Could you check a few things on this model? Use its own coordinates, in mm. Face numbers are marked on the shaded views. A direction names the side the tool comes from. Coordinates: 2 decimals unless noted, no trailing zeros. Loops run counter-clockwise (first coordinate to the right, second up) from the corner with the lowest first, then second, coordinate; pieces in that order, holes last.
from build123d import *

# Parameters (mm, degrees)
BOSS_EXTRUDE1_DEPTH = 215.9
BOSS_EXTRUDE2_DEPTH = 50.8
SKETCH4_W           = 19.05
SKETCH4_H           = 9.525
CUT_EXTRUDE1_DEPTH  = 31.1625
SKETCH3_R           = 3.175
BOSS_EXTRUDE3_DEPTH = 19.05


with BuildPart() as part:
    # Sketch1 → Boss-Extrude1 (new body, symmetric)
    with BuildSketch(Plane.XY):
        with BuildLine():
            Line((-19.05, -12.7), (19.05, -12.7))
            ThreePointArc((19.05, -12.7), (23.540128061, -10.840128061), (25.4, -6.35))
            Line((25.4, -6.35), (25.4, 6.35))
            ThreePointArc((25.4, 6.35), (23.540128061, 10.840128061), (19.05, 12.7))
            Line((19.05, 12.7), (-19.05, 12.7))
            ThreePointArc((-19.05, 12.7), (-23.540128061, 10.840128061), (-25.4, 6.35))
            Line((-25.4, 6.35), (-25.4, -6.35))
            ThreePointArc((-25.4, -6.35), (-23.540128061, -10.840128061), (-19.05, -12.7))
        make_face()
        with BuildLine():
            Line((-19.05, 11.049), (19.05, 11.049))
            ThreePointArc((19.05, 11.049), (22.372694765, 9.672694765), (23.749, 6.35))
            Line((23.749, 6.35), (23.749, -6.35))
            ThreePointArc((23.749, -6.35), (22.372694765, -9.672694765), (19.05, -11.049))
            Line((19.05, -11.049), (-19.05, -11.049))
            ThreePointArc((-19.05, -11.049), (-22.372694765, -9.672694765), (-23.749, -6.35))
            Line((-23.749, -6.35), (-23.749, 6.35))
            ThreePointArc((-23.749, 6.35), (-22.372694765, 9.672694765), (-19.05, 11.049))
        make_face(mode=Mode.SUBTRACT)
    extrude(amount=BOSS_EXTRUDE1_DEPTH, both=True)

    # Sketch2 → Boss-Extrude2 (add, through all)
    with BuildSketch(Plane(origin=(25.4, 0, 0), x_dir=(0, 0, -1), z_dir=(1, 0, 0))):
        with BuildLine():
            Line((203.2, -12.7), (203.2, -17.4625))
            Line((203.2, -17.4625), (220.6625, -17.4625))
            ThreePointArc((220.6625, -17.4625), (224.030096045, -9.332403955), (215.9, -12.7))
            Line((215.9, -12.7), (203.2, -12.7))
        make_face()
    extrude(amount=-BOSS_EXTRUDE2_DEPTH)

    # Sketch4 → Cut-Extrude1 (cut, through all)
    with BuildSketch(Plane.XZ.offset(17.4625)):
        with Locations((0, -220.6625)):
            Rectangle(SKETCH4_W, SKETCH4_H)
    extrude(amount=-CUT_EXTRUDE1_DEPTH, mode=Mode.SUBTRACT)

    # Sketch3 → Boss-Extrude3 (add, symmetric)
    with BuildSketch(Plane(origin=(0, 0, 0), x_dir=(0, 0, -1), z_dir=(1, 0, 0))):
        with Locations((220.6625, -12.7)):
            Circle(SKETCH3_R)
    extrude(amount=BOSS_EXTRUDE3_DEPTH, both=True)


solid = part.part
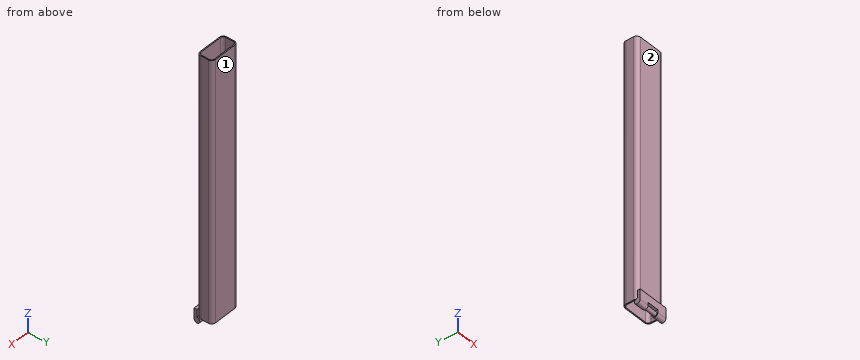
1) If I drill on L1, parallel to X at y = -4, z = -165; L2, parallel to Y at x = -10, z = 74; L3, parallel to Z at x = -0.5, y = -13, over which ranges is the centre line in solid material (lowest first)?
2) Imagine slicing it at A-A on z = 41. List the corners of the cut face in (x, y) for me, plus the area to 3 significant figures.
3) Will these pins go through, and if not, where does the flat tip stop? pin 1 (1.4 mm diameter, centred on x = -12.5, y = -15, fed in from +Z); pin 2 (19 mm diameter, centred on x = -3.5, z = 65, fed in from -Y); pin 3 (5 mm diameter, centred on x = -23, z = -210, fed in from +Y).
4) Imagine slicing it at B-B on x = -4. State how many separate pieces and enclosed holes the cut face has, plus the area to 3 significant figures.
5) For the marked faces 1 and 2, which set-ups out of +Z, -Z, +X, -X, +Y, -Y let a thin tool reach every point of the face, with its end or its side?
Solved:
1. L1: x = -25.4 to -23.75, 23.75 to 25.4
1. L2: y = -12.7 to -11.05, 11.05 to 12.7
1. L3: z = -223.82 to -217.5, -215.9 to -203.2
2. outline: (-25.4, -6.35) arc R6.35 ccw to (-19.05, -12.7) - (19.05, -12.7) arc R6.35 ccw to (25.4, -6.35) - (25.4, 6.35) arc R6.35 ccw to (19.05, 12.7) - (-19.05, 12.7) arc R6.35 ccw to (-25.4, 6.35) - close; hole (-23.75, -6.35) arc R4.7 ccw to (-19.05, -11.05) - (19.05, -11.05) arc R4.7 ccw to (23.75, -6.35) - (23.75, 6.35) arc R4.7 ccw to (19.05, 11.05) - (-19.05, 11.05) arc R4.7 ccw to (-23.75, 6.35) - close
2. area: 225 mm2
3. pin 1: stops at z = -203.2
3. pin 2: stops at y = -12.7
3. pin 3: stops at y = 12.53
4. separate pieces: 3
4. enclosed holes: 0
4. area: 1,520 mm2
5. face 1: +Z, -Z, +X, -X, +Y
5. face 2: +Z, +X, -X, -Y
